from build123d import *

# Parameters (mm, degrees)
SKETCH1_R               = 6.05
BOSS_EXTRUDE1_DEPTH     = 7.5
SKETCH2_R               = 2.5
BOSS_EXTRUDE2_DEPTH     = 11
CUT_EXTRUDE1_DEPTH      = 0.75
CUT_EXTRUDE1_DEPTH_BACK = 0.75
SKETCH3_W               = 22.1
SKETCH3_H               = 7.5
SKETCH4_R               = 0.625
CUT_EXTRUDE2_DEPTH      = 10
SKETCH5_R               = 3.5
CUT_EXTRUDE3_DEPTH      = 30.219043448
SKETCH6_R               = 1.5
CUT_EXTRUDE4_DEPTH      = 30.219043448


with BuildPart() as part:
    # Sketch1 → Boss-Extrude1 (new body)
    with BuildSketch(Plane.XY):
        with BuildLine():
            Line((-16.775, -7.286931796), (-2.615166667, -10.736079513))
            ThreePointArc((-2.615166667, -10.736079513), (11.05, 0), (-2.615166667, 10.736079513))
            Line((-2.615166667, 10.736079513), (-16.775, 7.286931796))
            ThreePointArc((-16.775, 7.286931796), (-22.5, 0), (-16.775, -7.286931796))
        make_face()
        Circle(SKETCH1_R, mode=Mode.SUBTRACT)
    extrude(amount=-BOSS_EXTRUDE1_DEPTH)

    # Sketch2 → Boss-Extrude2 (add)
    with BuildSketch(Plane.XY):
        with Locations((-15, 0)):
            Circle(SKETCH2_R)
    extrude(amount=BOSS_EXTRUDE2_DEPTH)

    # Sketch3 → Cut-Extrude1 (cut, two sides: drawn at the far end of the back side and taken through both)
    with BuildSketch(Plane(origin=(0, 0, 0), x_dir=(1, 0, 0), z_dir=(0, 1, 0)).offset(-CUT_EXTRUDE1_DEPTH_BACK)):
        with Locations((11.05, 3.75)):
            Rectangle(SKETCH3_W, SKETCH3_H)
    extrude(amount=CUT_EXTRUDE1_DEPTH + CUT_EXTRUDE1_DEPTH_BACK, mode=Mode.SUBTRACT)

    # Sketch4 → Cut-Extrude2 (cut)
    with BuildSketch(Plane.XY.offset(11)):
        with Locations((-15, 0)):
            Circle(SKETCH4_R)
    extrude(amount=-CUT_EXTRUDE2_DEPTH, mode=Mode.SUBTRACT)

    # Sketch5 → Cut-Extrude3 (cut, through all)
    with BuildSketch(Plane(origin=(0, 4, 0), x_dir=(1, 0, 0), z_dir=(0, 1, 0))):
        with Locations((8.513925269, 3.75)):
            Circle(SKETCH5_R)
    extrude(amount=CUT_EXTRUDE3_DEPTH, mode=Mode.SUBTRACT)

    # Sketch6 → Cut-Extrude4 (cut, through all)
    with BuildSketch(Plane(origin=(0, 4, 0), x_dir=(1, 0, 0), z_dir=(0, 1, 0))):
        with Locations(Location((8.513925269, 3.75, 0), (0, 0, 270))):
            Circle(SKETCH6_R)
    extrude(amount=-CUT_EXTRUDE4_DEPTH, mode=Mode.SUBTRACT)


solid = part.part
Here's how the part is built. I have some questions about the finished solid (model axes, mm). A direction names the side the tool comes from. Round coordinates to 2 decimals unless told otherwise and drop trailing zeros. Order: outer loops, then holes, each group sorted by start corner. A loop starts at its lowest first (then second) coordinate and runs counter-clockwise, first axis right, second up. Notation, with made-up numbers: M 2.25,49 L 53.25,49 A17 ccw 53.25,65 Z; hole C -18,62 d11. An arc over 180 degrees is marked long. Return JSON: item names as keys, results as strings. Group by question number.
1. On a 3-axis mill with a long thin cutter (end or side, diameter ignored), from which of +Z, -Z, +X, -X, +Y, -Y can I reach the whole of each face in a straight line? I mean faces 5 (the face through (-6, -2, -7.5)), 6 (the face through (8.5, -0.75, -5.5)), 7 (the face through (-17.5, 0.1, 5.4)), 8 (the face through (5.015, 6.233, -3.853)). Say none if no direction works.
2. I'm going to push flat-ended pins straight in: pin 1 Ø5.5 at (x, z) = (9, -5) entering from -Y; pin 2 Ø0.6 at (x, y) = (-15, 0) entering from +Z; pin 3 Ø6 at (x, z) = (8, -4) entering from +Y; pin 4 Ø1.5 at (y, z) = (3.5, 4.5) entering from -X. Where does each tip first touch, or does it pass through?
3. If we section it at B-B on y = -1.5: List the corners of the cut face in (x, z) for me, then the cut area to 3 significant figures.
4. If we mould it in two halves opening along Z, with no side actions, what happens to faces 1 (the face through (7.05, -3.72, -4.08)), 2 (the face through (7, 4, -3)), 3 (the face through (-9.79, -8.99, -3.7)), 4 (the face through (-6, -2, 0))? For each: pulls with the +Z half, pulls with the -Z half, needs draft (parallel to the pull), parting line crosses it, or undercut.
5. If we section it at D-D on y = 5.25: List the corners of the cut face in (x, z) for me, then the cut area to 3 significant figures.
6. If we section it at A-A on x = 0: List the corners of the cut face in (y, z) for me.
7. Please list where these lines run through material, in increasing order: probe 1 along Y at (x, z) = (-15, 8.5) (3 decimals); probe 2 along Y at (x, z) = (0, -2.25); probe 3 along X at (y, z) = (-3.5, -3.75).
8. If we section it at C-C on z = -3.75: List the corners of the cut face in (x, y) for me (3 decimals).
Reply:
{
 "1": {"face 5": "-Z, +X, -X, +Y, -Y", "face 6": "+Z, -Z, +X", "face 7": "+Z", "face 8": "+Y"},
 "2": {"pin 1": "y = -9.11", "pin 2": "z = 1", "pin 3": "y = 9.85", "pin 4": "through"},
 "3": {"outline": "M -22.35,-7.5 L -5.86,-7.5 L -5.86,0 L -13,0 L -13,11 L -17,11 L -17,0 L -22.35,0 Z; M 5.86,-7.5 L 10.95,-7.5 L 10.95,0 L 5.86,0 Z; hole C 8.51,-3.75 d3", "area": "199 mm^2"},
 "4": {"face 1": "undercut", "face 2": "undercut", "face 3": "needs draft", "face 4": "pulls with the +Z half"},
 "5": {"outline": "M -20.36,-7.5 L -3.01,-7.5 L -3.01,0 L -20.36,0 Z; M 3.01,-7.5 L 9.72,-7.5 L 9.72,-7.03 A3.5 cw long 9.72,-0.47 L 9.72,0 L 3.01,0 Z", "area": "153 mm^2"},
 "6": {"outline": "M -11.05,-7.5 L -6.05,-7.5 L -6.05,0 L -11.05,0 Z; M 6.05,-7.5 L 11.05,-7.5 L 11.05,0 L 6.05,0 Z"},
 "7": {"probe 1": "-2.5 to -0.625, 0.625 to 2.5", "probe 2": "-11.05 to -6.05, 6.05 to 11.05", "probe 3": "-21.63 to -4.93, 4.93 to 7.01, 10.01 to 10.48"},
 "8": {"outline": "M -16.775,-7.287 L -2.615,-10.736 A11.05 ccw 7.014,-8.539 L 7.014,-0.75 L 6.003,-0.75 A6.05 cw long 6.003,0.75 L 7.014,0.75 L 7.014,4 L 5.014,4 L 5.014,9.847 A11.05 ccw -2.615,10.736 L -16.775,7.287 A7.5 ccw Z; M 10.014,-4.672 A11.05 ccw 11.025,-0.75 L 10.014,-0.75 Z; M 10.014,0.75 L 11.025,0.75 A11.05 ccw 10.301,4 L 10.014,4 Z"}
}
